Check sheet for the drawn part. Datum: minimum x, y, z corner. Units: mm. A direction names the side the tool comes from. Give positions to 0.01 mm unless a question says otherwise; leave off trailing zeros. Loops run counter-clockwise (first coordinate to the right, second up) from the corner with the lowest first, then second, coordinate; pieces in that order, holes last.
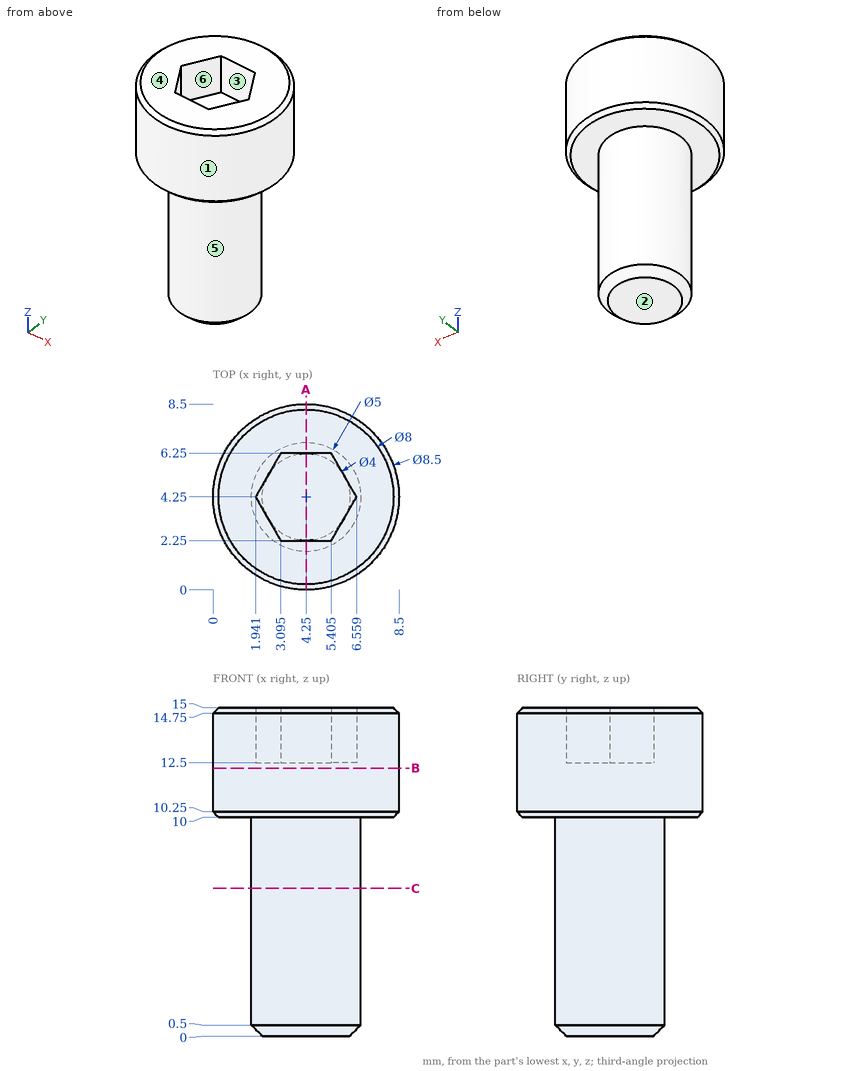
1) Sectioned sample at B-B on z = 12.25. Enter the section's corners in (x, y).
2) Scan lines: line 1 along Z through (x, y) = (3, 7.5); line 2 along Y through (x, z) = (3.5, 14.25); line 3 along Z through (x, y) = (3.5, 3). Record each from-to range of solid material in increasing order.
3) Sectioned sample at C-C on z = 6.75. Enter the section's corners in (x, y), plus the area to 3 significant figures.
4) Tool access check on the marked faces 4, 5 and 6. Record the directions out of +Z, -Z, +X, -X, +Y, -Y that give a thin tool (end or side, any length) a straight path to the whole face; none if there is none.
5) Sectioned sample at A-A on x = 4.25. Enter the section's corners in (y, z).
6) Depth check by flat-ended pin: P1, Ø4, axis at x = 5, y = 5, coming from the -Z side; P2, Ø1.5, axis at y = 1.5, z = 3, coming from the +X side; P3, Ø1.5, axis at x = 4.5, z = 9, coming from the +Y side. Enter the tip coordinate at first touch or a pass-through.
7) Mould release check, pull along Y, two halves, no side actions. Record for the marked faces 1, 2 and 3: +Y half, -Y half, draft (parallel to the pull), parting line (faces both ways), or undercut.
Determined:
1. outline: circle Ø8.5 at (4.25, 4.25)
2. line 1: z = 10 to 15
2. line 2: y = 0.07 to 2.25, 6.25 to 8.43
2. line 3: z = 0 to 12.5
3. outline: circle Ø5 at (4.25, 4.25)
3. area: 19.6 mm2
4. face 4: +Z, +X, -X, +Y, -Y
4. face 5: -Z
4. face 6: +Z
5. outline: (0, 10.25) - (0.25, 10) - (1.75, 10) - (1.75, 0.5) - (2.25, 0) - (6.25, 0) - (6.75, 0.5) - (6.75, 10) - (8.25, 10) - (8.5, 10.25) - (8.5, 14.75) - (8.25, 15) - (6.25, 15) - (6.25, 12.5) - (2.25, 12.5) - (2.25, 15) - (0.25, 15) - (0, 14.75) - close
6. P1: stops at z = 0
6. P2: stops at x = 5.75
6. P3: stops at y = 6.75
7. face 1: parting line
7. face 2: draft
7. face 3: undercut
